```python
from build123d import *

# Parameters (mm, degrees)
SKETCH1_W           = 510
SKETCH1_H           = 305
SKETCH1_W_2         = 500
SKETCH1_H_2         = 295
BOSS_EXTRUDE1_DEPTH = 120
SKETCH2_W           = 510
SKETCH2_H           = 305
BOSS_EXTRUDE2_DEPTH = 2
SKETCH3_W           = 510
SKETCH3_H           = 305
BOSS_EXTRUDE3_DEPTH = 2
CUT_EXTRUDE1_DEPTH  = 306
SKETCH5_W           = 490
SKETCH5_H           = 285
CUT_EXTRUDE4_DEPTH  = 125
CUT_EXTRUDE5_DEPTH  = 511


with BuildPart() as part:
    # Sketch1 → Boss-Extrude1 (new body)
    with BuildSketch(Plane(origin=(0, 0, 0), x_dir=(0, 0, -1), z_dir=(1, 0, 0))):
        with Locations((250, 147.5)):
            Rectangle(SKETCH1_W, SKETCH1_H)
        with Locations((250, 147.5)):
            Rectangle(SKETCH1_W_2, SKETCH1_H_2, mode=Mode.SUBTRACT)
    extrude(amount=BOSS_EXTRUDE1_DEPTH)

    # Sketch2 → Boss-Extrude2 (add)
    with BuildSketch(Plane(origin=(120, 0, 0), x_dir=(0, 0, -1), z_dir=(1, 0, 0))):
        with Locations((250, 147.5)):
            Rectangle(SKETCH2_W, SKETCH2_H)
    extrude(amount=BOSS_EXTRUDE2_DEPTH)

    # Sketch3 → Boss-Extrude3 (add)
    with BuildSketch(Plane.ZY):
        with Locations((-250, 147.5)):
            Rectangle(SKETCH3_W, SKETCH3_H)
    extrude(amount=BOSS_EXTRUDE3_DEPTH)

    # Sketch4 → Cut-Extrude1 (cut, through all)
    with BuildSketch(Plane.XZ.offset(5)):
        Polygon((14.260678291, -495), (112, -365.295539257), (112, -495), align=None)
        Polygon((73.092374529, -400.311300748), (8, -351.260678291), (8, -486.691799294), align=None)
        Polygon((79.110524761, -392.324945648), (112, -348.679137846), (112, -218.265533068), (13.582159118, -342.945780321), align=None)
        Polygon((8, -333.877817445), (112, -202.125834287), (112, -5), (8, -5), align=None)
    extrude(amount=-CUT_EXTRUDE1_DEPTH, mode=Mode.SUBTRACT)

    # Sketch5 → Cut-Extrude4 (cut, through all)
    with BuildSketch(Plane.ZY.offset(2)):
        with Locations((-250, 147.5)):
            Rectangle(SKETCH5_W, SKETCH5_H)
    extrude(amount=-CUT_EXTRUDE4_DEPTH, mode=Mode.SUBTRACT)

    # Sketch8 → Cut-Extrude5 (cut, through all)
    with BuildSketch(Plane.XY.offset(5)):
        Polygon((15.640858332, 5), (112, 88.387718751), (112, 5), align=None)
        Polygon((70.792299268, 65.951771), (8, 138.511761264), (8, 11.612281249), align=None)
        Polygon((78.353986092, 222.504461556), (112, 193.387718751), (112, 101.612281249), (78.353986092, 72.495538444), (13.446278977, 147.5), align=None)
        Polygon((70.792299268, 229.048229), (8, 156.488238736), (8, 283.387718751), align=None)
        Polygon((15.640858332, 290), (112, 206.612281249), (112, 290), align=None)
    extrude(amount=-CUT_EXTRUDE5_DEPTH, mode=Mode.SUBTRACT)


solid = part.part
```
Read the model definition and answer for the solid it produces. Units are mm, in the model's axes. A direction names the side the tool comes from. Give positions to 0.01 mm unless a question says otherwise; leave off trailing zeros. Order: outer loops, then holes, each group sorted by start corner. A loop starts at its lowest first (then second) coordinate and runs counter-clockwise, first axis right, second up.
(1) Find section B-B (y = 200.5). Give the number of separate pieces and of enclosed holes in the cut face, plus the area to 3 significant figures.
(2) Straight lines are drawn through the part: L1, parallel to Y at x = 114.5, z = -379.5; L2, parallel to Z at x = 7, y = 95. For each, find the intervals that lie inside material, in ascending order.
(3) Find section A-A (z = -81.5). Give the vertices of the cut face in (x, y).
(4) For faces 1 (the flat face through (33, 124, -505)), 2 (the flat face through (41, 297.46, -376.13)), 3 (the flat face through (120, 290.2, -248.8)), 4 (the flat face through (94.94, 208.15, 2.54)), determine the directions among +Z, -Z, +X, -X, +Y, -Y from which every point of the face is accessible in a straight line to the end or side of a thin tool.
(5) For a pull along X with two mould halves and no side action, classify faces 5 (the flat face through (-2, 1, -327)), 6 (the flat face through (55.7, 300, -289)), 7 (the flat face through (38.957, 256.598, -502.465)) as released by +X, released by -X, zero draft, split by the parting line, or undercut.
Result sheet:
1. separate pieces: 6
1. enclosed holes: 0
1. area: 454 mm2
2. L1: y = -5 to 0, 295 to 300
2. L2: z = -505 to -500, 0 to 5
3. outline: (-2, -5) - (8, -5) - (8, 0) - (0, 0) - (0, 5) - (-2, 5) - close; (-2, 290) - (0, 290) - (0, 295) - (8, 295) - (8, 300) - (-2, 300) - close; (112, -5) - (122, -5) - (122, 5) - (120, 5) - (120, 0) - (112, 0) - close; (112, 295) - (120, 295) - (120, 290) - (122, 290) - (122, 300) - (112, 300) - close
4. face 1: -Z, +X, -X, +Y, -Y
4. face 2: +Y, -Y
4. face 3: none
4. face 4: +Z, -Z
5. face 5: released by -X
5. face 6: zero draft
5. face 7: undercut
